Work out the finished part from the listing and answer in its coordinate system (mm). Face numbers are marked on the shaded views. A direction names the side the tool comes from. Coordinates: 2 decimals unless noted, no trailing zeros. Order: outer loops, then holes, each group sorted by start corner. A loop starts at its lowest first (then second) coordinate and runs counter-clockwise, first axis right, second up. Notation, with made-up numbers: M 82,7 L 115,7 A22 cw 115,26 Z; hole C 83.25,37 d5. An arc over 180 degrees is marked long. Answer in a Markdown table with one row per item. Add a question column.
Item 1: The part is cut by section D-D (x = 18). Write down the section's boundary in (y, z), then the cut area to 3 significant figures.
Item 2: Flat-ended cylindrical pins translate along their axes: pin 1 Ø6 at (y, z) = (7, 21) entering from -X; pin 2 Ø3.5 at (x, z) = (-2, 14) entering from -Y; pin 3 Ø7 at (x, z) = (18, 14) entering from -Y; pin 4 Ø3.5 at (y, z) = (17.5, 34) entering from -X. Find the tip coordinate at first contact, or state that the pin passes through.
Item 3: The part is cut by section A-A (z = 34). Write down the section's boundary in (x, y).
Item 4: Consider line 1 (X direction, y = 24, z = 14); line 2 (Z direction, x = 3.5, y = 9); line 3 (Z direction, x = -2, y = 25). Determine where each line is inside the solid, lowest interval first. Write a range as from..to.
Item 5: The mould has two halves that part along Z. Classify the marked faces 4, 5 and 6: released by +Z, released by -Z, zero draft, split by the parting line, or undercut.
Item 6: The part is cut by section C-C (y = 4). Write down the section's boundary in (x, z).
Item 7: The part is cut by section B-B (x = -21). Write down the section's boundary in (y, z), then the cut area to 3 significant figures.
Item 8: Which of the six approach directions +Z, -Z, +X, -X, +Y, -Y give full straight-line access (tool end or side, diameter ignored) to the marked faces 1, 2 and 3?
from build123d import *

# Parameters (mm, degrees)
BOSS_EXTRUDE1_DEPTH     = 28
BOSS_EXTRUDE2_DEPTH     = 12
SKETCH3_R               = 2.25
CUT_EXTRUDE1_DEPTH      = 62.565006294
SKETCH4_R               = 2.25
CUT_EXTRUDE2_DEPTH      = 56.554027757
SKETCH5_W               = 40
SKETCH5_H               = 5
BOSS_EXTRUDE3_DEPTH     = 25
CUT_EXTRUDE3_DEPTH      = 10
CUT_EXTRUDE3_DEPTH_BACK = 54.209491634
SKETCH6_R               = 2.25
SKETCH7_W               = 7
SKETCH7_H               = 5
CUT_EXTRUDE4_DEPTH      = 10
SKETCH8_R               = 2.25
BOSS_EXTRUDE4_DEPTH     = 8
BOSS_EXTRUDE6_DEPTH     = 4
SKETCH10_W              = 8
SKETCH10_H              = 28
CUT_EXTRUDE5_DEPTH      = 66.423619588


with BuildPart() as part:
    # Sketch1 → Boss-Extrude1 (new body)
    with BuildSketch(Plane(origin=(0, 0, 0), x_dir=(1, 0, 0), z_dir=(0, 1, 0))):
        Polygon((0, 0), (-26.5, 0), (-26.5, 10), (-10, 10), (-10, 40), (0, 40), align=None)
    extrude(amount=BOSS_EXTRUDE1_DEPTH)

    # Sketch2 → Boss-Extrude2 (add)
    with BuildSketch(Plane.ZY.offset(26.5)):
        with BuildLine():
            Line((0, 28), (0, 0))
            Line((0, 0), (8, 0))
            Line((8, 0), (8, 8))
            ThreePointArc((8, 8), (4, 12), (8, 16))
            Line((8, 16), (8, 28))
            Line((8, 28), (0, 28))
        make_face()
    extrude(amount=-BOSS_EXTRUDE2_DEPTH)

    # Sketch3 → Cut-Extrude1 (cut, through all)
    with BuildSketch(Plane.XY.offset(8)):
        with Locations((-20.5, 20)):
            Circle(SKETCH3_R)
        with Locations((-20.5, 4)):
            Circle(SKETCH3_R)
    extrude(amount=-CUT_EXTRUDE1_DEPTH, mode=Mode.SUBTRACT)

    # Sketch4 → Cut-Extrude2 (cut, through all)
    with BuildSketch(Plane(origin=(0, 0, 0), x_dir=(0, 0, -1), z_dir=(1, 0, 0))):
        with Locations((34, 17.5)):
            Circle(SKETCH4_R)
    extrude(amount=-CUT_EXTRUDE2_DEPTH, mode=Mode.SUBTRACT)

    # Sketch5 → Boss-Extrude3 (add)
    with BuildSketch(Plane(origin=(0, 0, 0), x_dir=(0, 0, -1), z_dir=(1, 0, 0))):
        with Locations((20, 25.5)):
            Rectangle(SKETCH5_W, SKETCH5_H)
    extrude(amount=BOSS_EXTRUDE3_DEPTH)

    # Sketch6 → Cut-Extrude3 (cut, two sides: drawn at the far end of the back side and taken through both)
    with BuildSketch(Plane.XZ.offset(-23).offset(-CUT_EXTRUDE3_DEPTH_BACK)):
        with Locations(Location((-2, -14, 0), (0, 0, 332.733955549))):
            Circle(SKETCH6_R)
        with Locations(Location((18, -14, 0), (0, 0, 90))):
            Circle(SKETCH6_R)
    extrude(amount=CUT_EXTRUDE3_DEPTH + CUT_EXTRUDE3_DEPTH_BACK, mode=Mode.SUBTRACT)

    # Sketch7 → Cut-Extrude4 (cut)
    with BuildSketch(Plane(origin=(0, 0, 0), x_dir=(0, 0, -1), z_dir=(1, 0, 0))):
        with Locations((14, 20.5)):
            Rectangle(SKETCH7_W, SKETCH7_H)
    extrude(amount=-CUT_EXTRUDE4_DEPTH, mode=Mode.SUBTRACT)

    # Sketch8 → Boss-Extrude4 (add)
    with BuildSketch(Plane.XY):
        with BuildLine():
            Line((-9.5, -9), (-4.52228171, -15.720105701))
            ThreePointArc((-4.52228171, -15.720105701), (1.041905897, -18.22646272), (6.089442895, -14.796538598))
            Line((6.089442895, -14.796538598), (25, 23))
            Line((25, 23), (0, 23))
            Line((0, 23), (0, 0))
            Line((0, 0), (-26.5, 0))
            Line((-26.5, 0), (-10.922493011, -7.804616818))
            ThreePointArc((-10.922493011, -7.804616818), (-10.14087473, -8.318566759), (-9.5, -9))
        make_face()
        with Locations((0.5, -12)):
            Circle(SKETCH8_R, mode=Mode.SUBTRACT)
    extrude(amount=-BOSS_EXTRUDE4_DEPTH)

    # Sketch9 → Boss-Extrude6 (add)
    with BuildSketch(Plane(origin=(0, 0, -40), x_dir=(-1, 0, 0), z_dir=(0, 0, -1))):
        Polygon((-25, 23), (0, 0), (10, 0), (10, 28), (-25, 28), align=None)
    extrude(amount=BOSS_EXTRUDE6_DEPTH)

    # Sketch10 → Cut-Extrude5 (cut, through all)
    with BuildSketch(Plane(origin=(-14.5, 0, 0), x_dir=(0, 0, -1), z_dir=(1, 0, 0))):
        with Locations((-4, 14)):
            Rectangle(SKETCH10_W, SKETCH10_H)
    extrude(amount=-CUT_EXTRUDE5_DEPTH, mode=Mode.SUBTRACT)


with BuildPart() as body_2:
    # Mirror1: mirrored copy
    add(part.part.mirror(Plane(origin=(0, 28, 0), x_dir=(1, 0, 0), z_dir=(0, 0, -1))))


solid = body_2.part
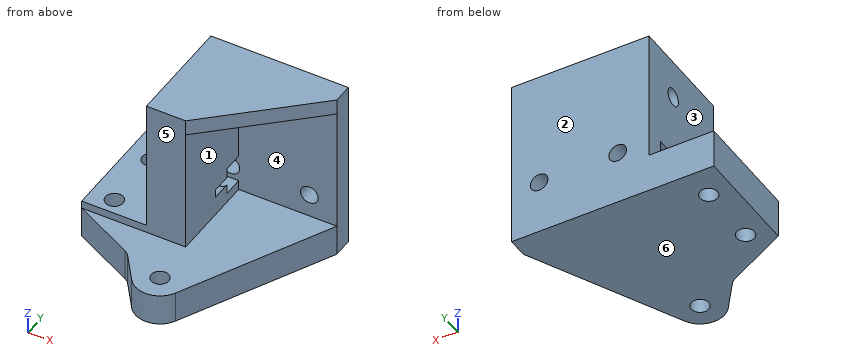
Reply:
| question | item | result |
|---|---|---|
| 1 | outline | M 9.01,0 L 28,0 L 28,11.75 L 23,11.75 L 23,8 L 9.01,8 Z; M 16.56,40 L 23,40 L 23,16.25 L 28,16.25 L 28,44 L 16.56,44 Z |
| 1 | area | 335 mm2 |
| 2 | pin 1 | stops at x = -10 |
| 2 | pin 2 | stops at y = 0 |
| 2 | pin 3 | stops at y = 23 |
| 2 | pin 4 | passes through |
| 3 | outline | M -10,0 L 0,0 L 0,15.25 L -10,15.25 Z; M -10,19.75 L 0,19.75 L 0,23 L 25,23 L 25,28 L -10,28 Z |
| 4 | line 1 | x = -10..-4.25, 0.25..15.75, 20.25..25 |
| 4 | line 2 | z = 0..8, 40..44 |
| 4 | line 3 | z = 0..11.75, 16.25..44 |
| 5 | face 4 | undercut |
| 5 | face 5 | zero draft |
| 5 | face 6 | released by -Z |
| 6 | outline | M -26.5,0 L -22.75,0 L -22.75,10 L -26.5,10 Z; M -18.25,0 L 15.49,0 L 15.49,8 L 0,8 L 0,40 L 4.35,40 L 4.35,44 L -10,44 L -10,10 L -18.25,10 Z |
| 7 | outline | M -2.76,0 L 1.81,0 L 1.81,10 L 0,10 L 0,8 L -2.76,8 Z; M 6.19,0 L 17.81,0 L 17.81,10 L 6.19,10 Z; M 22.19,0 L 28,0 L 28,10 L 22.19,10 Z |
| 7 | area | 214 mm2 |
| 8 | face 1 | +X, -Y |
| 8 | face 2 | +Z, -Z, +X, -X, +Y |
| 8 | face 3 | +Z, -X, +Y, -Y |
